```python
from build123d import *

# Parameters (mm, degrees)
BOX002_W      = 10
BOX002_H      = 4
BOX002_DEPTH  = 13
BOX003_W      = 10
BOX003_H      = 4
BOX003_DEPTH  = 13
BOX004_W      = 10
BOX004_H      = 4
BOX004_DEPTH  = 13
BOX005_W      = 10
BOX005_H      = 4
BOX005_DEPTH  = 13
BOX006_W      = 19
BOX006_H      = 4
BOX006_DEPTH  = 15
BOX007_W      = 4
BOX007_H      = 12
BOX007_DEPTH  = 3
BOX008_W      = 4
BOX008_H      = 12
BOX008_DEPTH  = 3
BOX001_W      = 10
BOX001_H      = 4
BOX001_DEPTH  = 13
BOX_W         = 100
BOX_H         = 55
BOX_DEPTH     = 2
TUBE_R        = 4
TUBE_R_2      = 1.9
TUBE_DEPTH    = 6
TUBE001_R     = 4
TUBE001_R_2   = 1.9
TUBE001_DEPTH = 6
TUBE002_R     = 4
TUBE002_R_2   = 1.9
TUBE002_DEPTH = 6
TUBE003_R     = 4
TUBE003_R_2   = 1.9
TUBE003_DEPTH = 6
SKETCH_W      = 99
SKETCH_H      = 54
PAD_DEPTH     = 30


with BuildPart() as barrelcutout001:
    # Box002 → Box002 (new body)
    with BuildSketch(Plane(origin=(53, 52, 7), x_dir=(1, 0, 0), z_dir=(0, 0, 1))):
        with Locations((5, 2)):
            Rectangle(BOX002_W, BOX002_H)
    extrude(amount=BOX002_DEPTH)


with BuildPart() as barrelcutout002:
    # Box003 → Box003 (new body)
    with BuildSketch(Plane(origin=(35, 52, 7), x_dir=(1, 0, 0), z_dir=(0, 0, 1))):
        with Locations((5, 2)):
            Rectangle(BOX003_W, BOX003_H)
    extrude(amount=BOX003_DEPTH)


with BuildPart() as barrelcutout003:
    # Box004 → Box004 (new body)
    with BuildSketch(Plane(origin=(17, 52, 7), x_dir=(1, 0, 0), z_dir=(0, 0, 1))):
        with Locations((5, 2)):
            Rectangle(BOX004_W, BOX004_H)
    extrude(amount=BOX004_DEPTH)


with BuildPart() as barrelcutout004:
    # Box005 → Box005 (new body)
    with BuildSketch(Plane(origin=(71, -3, 7), x_dir=(1, 0, 0), z_dir=(0, 0, 1))):
        with Locations((5, 2)):
            Rectangle(BOX005_W, BOX005_H)
    extrude(amount=BOX005_DEPTH)


with BuildPart() as obj1:
    # Box006 → Box006 (new body)
    with BuildSketch(Plane(origin=(49.5, -3, 7), x_dir=(1, 0, 0), z_dir=(0, 0, 1))):
        with Locations((9.5, 2)):
            Rectangle(BOX006_W, BOX006_H)
    extrude(amount=BOX006_DEPTH)


with BuildPart() as latchcut:
    # Box007 → Box007 (new body)
    with BuildSketch(Plane(origin=(-2.5, 21, 25.5), x_dir=(1, 0, 0), z_dir=(0, 0, 1))):
        with Locations((2, 6)):
            Rectangle(BOX007_W, BOX007_H)
    extrude(amount=BOX007_DEPTH)


with BuildPart() as latchcut001:
    # Box008 → Box008 (new body)
    with BuildSketch(Plane(origin=(97.5, 21, 25.5), x_dir=(1, 0, 0), z_dir=(0, 0, 1))):
        with Locations((2, 6)):
            Rectangle(BOX008_W, BOX008_H)
    extrude(amount=BOX008_DEPTH)


with BuildPart() as cuts:
    # Box001 → Box001 (new body)
    with BuildSketch(Plane(origin=(71, 52, 7), x_dir=(1, 0, 0), z_dir=(0, 0, 1))):
        with Locations((5, 2)):
            Rectangle(BOX001_W, BOX001_H)
    extrude(amount=BOX001_DEPTH)

    # Fusion001: union BarrelCutout001, BarrelCutout002, BarrelCutout003, BarrelCutout004, obj1, LatchCut, LatchCut001
    add(barrelcutout001.part)
    add(barrelcutout002.part)
    add(barrelcutout003.part)
    add(barrelcutout004.part)
    add(obj1.part)
    add(latchcut.part)
    add(latchcut001.part)


with BuildPart() as base:
    # Box → Box (new body)
    with BuildSketch(Plane(origin=(-0.5, -0.5, 0), x_dir=(1, 0, 0), z_dir=(0, 0, 1))):
        with Locations((50, 27.5)):
            Rectangle(BOX_W, BOX_H)
    extrude(amount=BOX_DEPTH)


with BuildPart() as standoff:
    # Tube → Tube (new body)
    with BuildSketch(Plane(origin=(7, 7, 0), x_dir=(1, 0, 0), z_dir=(0, 0, 1))):
        Circle(TUBE_R)
        Circle(TUBE_R_2, mode=Mode.SUBTRACT)
    extrude(amount=TUBE_DEPTH)


with BuildPart() as standoff001:
    # Tube001 → Tube001 (new body)
    with BuildSketch(Plane(origin=(92, 7, 0), x_dir=(1, 0, 0), z_dir=(0, 0, 1))):
        Circle(TUBE001_R)
        Circle(TUBE001_R_2, mode=Mode.SUBTRACT)
    extrude(amount=TUBE001_DEPTH)


with BuildPart() as standoff002:
    # Tube002 → Tube002 (new body)
    with BuildSketch(Plane(origin=(7, 47, 0), x_dir=(1, 0, 0), z_dir=(0, 0, 1))):
        Circle(TUBE002_R)
        Circle(TUBE002_R_2, mode=Mode.SUBTRACT)
    extrude(amount=TUBE002_DEPTH)


with BuildPart() as standoff003:
    # Tube003 → Tube003 (new body)
    with BuildSketch(Plane(origin=(92, 47, 0), x_dir=(1, 0, 0), z_dir=(0, 0, 1))):
        Circle(TUBE003_R)
        Circle(TUBE003_R_2, mode=Mode.SUBTRACT)
    extrude(amount=TUBE003_DEPTH)


with BuildPart() as obj2:
    # Sketch → Pad (new body)
    with BuildSketch(Plane.XY):
        with BuildLine():
            ThreePointArc((0, 56), (-1.414214, 55.414214), (-2, 54))
            Line((-2, 0), (-2, 54))
            ThreePointArc((-2, 0), (-1.414214, -1.414214), (0, -2))
            Line((99, -2), (0, -2))
            ThreePointArc((99, -2), (100.414214, -1.414214), (101, 0))
            Line((101, 54), (101, 0))
            ThreePointArc((101, 54), (100.414207, 55.41422), (98.999983, 56))
            Line((0, 56), (98.999983, 56))
        make_face()
        with Locations((49.5, 27)):
            Rectangle(SKETCH_W, SKETCH_H, mode=Mode.SUBTRACT)
    extrude(amount=PAD_DEPTH)

    # Fusion: union Base, Standoff, Standoff001, Standoff002, Standoff003
    add(base.part)
    add(standoff.part)
    add(standoff001.part)
    add(standoff002.part)
    add(standoff003.part)

    # Cut: cut Cuts
    add(cuts.part, mode=Mode.SUBTRACT)


solid = obj2.part
```
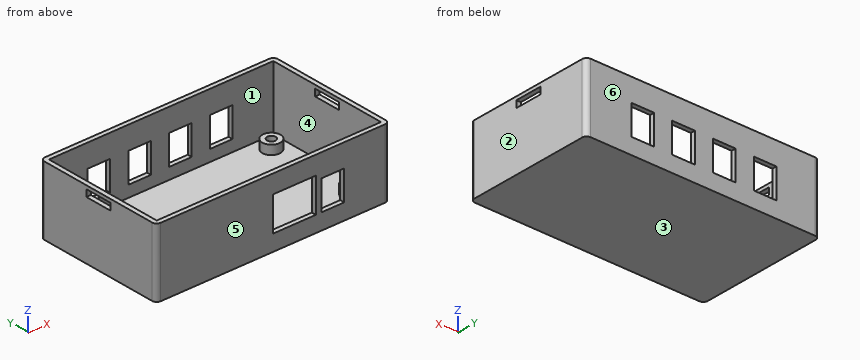
Verification items for the finished model (mm, model axes). Face numbers are marked on the shaded views. A direction names the side the tool comes from. Round coordinates to 2 decimals unless told otherwise and drop trailing zeros. Order: outer loops, then holes, each group sorted by start corner. A loop starts at its lowest first (then second) coordinate and runs counter-clockwise, first axis right, second up. Notation, with made-up numbers: (79.25, -23.5) -> (91.25, -23.5) arc R29 ccw to (91.25, 0.5) -> close; hole circle Ø11 at (-24, 23.25). An arc over 180 degrees is marked (long way). Put each result on its own line as item: value. Start each with the question number.
(1) Draft check along Y on the marked faces 3, 4, 5 and 6. Enter one of: +Y half, -Y half, draft (parallel to the pull), parting line (faces both ways), or undercut.
(2) Section check C-C (z = 9.25). State how many separate pieces and enclosed holes the cut face has, then the cut area to 3 significant figures.
(3) Depth check by flat-ended pin: pin 1 Ø2.5 at (x, y) = (90.5, 9) entering from +Z; pin 2 Ø6 at (x, y) = (39, 14.5) entering from +Z; pin 3 Ø1 at (x, z) = (-1, 27.5) entering from +Y. Enter the tip coordinate at first touch or a pass-through.
(4) Section check A-A (y = 25.5). Enter the section's corners in (x, z), then the cut area to 3 significant figures.
(5) Section check D-D (x = 92). Enter the section's corners in (y, z).
(6) Material ranges on line 1 along Y through (x, z) = (7, 5); line 2 along X through (y, z) = (47, 4.1); line 3 along X through (y, z) = (7, 19.75), recorded low to high.
(7) Tool access check on the marked faces 1 and 2. Record the directions out of +Z, -Z, +X, -X, +Y, -Y that give a thin tool (end or side, any length) a straight path to the whole face; none if there is none.
(8) Section check B-B (y = 7). Enter the section's corners in (x, z).
Completed:
1. face 3: draft
1. face 4: undercut
1. face 5: -Y half
1. face 6: +Y half
2. separate pieces: 6
2. enclosed holes: 0
2. area: 487 mm2
3. pin 1: stops at z = 6
3. pin 2: stops at z = 2
3. pin 3: stops at y = 55.94
4. outline: (-2, 0) -> (101, 0) -> (101, 25.5) -> (99, 25.5) -> (99, 2) -> (0, 2) -> (0, 25.5) -> (-2, 25.5) -> close; (-2, 28.5) -> (0, 28.5) -> (0, 30) -> (-2, 30) -> close; (99, 28.5) -> (101, 28.5) -> (101, 30) -> (99, 30) -> close
4. area: 306 mm2
5. outline: (-2, 0) -> (56, 0) -> (56, 30) -> (54, 30) -> (54, 2) -> (51, 2) -> (51, 6) -> (48.9, 6) -> (48.9, 2) -> (45.1, 2) -> (45.1, 6) -> (43, 6) -> (43, 2) -> (11, 2) -> (11, 6) -> (8.9, 6) -> (8.9, 2) -> (5.1, 2) -> (5.1, 6) -> (3, 6) -> (3, 2) -> (0, 2) -> (0, 30) -> (-2, 30) -> close
6. line 1: y = -2 to 0, 3 to 5.1, 8.9 to 11, 43 to 45.1, 48.9 to 51, 54 to 56
6. line 2: x = -2 to 0, 3 to 5.1, 8.9 to 11, 88 to 90.1, 93.9 to 96, 99 to 101
6. line 3: x = -2 to 0, 99 to 101
7. face 1: +Z
7. face 2: +Z, -Z, +X, +Y, -Y
8. outline: (-2, 0) -> (101, 0) -> (101, 30) -> (99, 30) -> (99, 2) -> (96, 2) -> (96, 6) -> (93.9, 6) -> (93.9, 2) -> (90.1, 2) -> (90.1, 6) -> (88, 6) -> (88, 2) -> (11, 2) -> (11, 6) -> (8.9, 6) -> (8.9, 2) -> (5.1, 2) -> (5.1, 6) -> (3, 6) -> (3, 2) -> (0, 2) -> (0, 30) -> (-2, 30) -> close
